Read the model definition and answer for the solid it produces. Units are mm, in the model's axes. Face numbers are marked on the shaded views. A direction names the side the tool comes from. Coordinates: 2 decimals unless noted, no trailing zeros. Loops run counter-clockwise (first coordinate to the right, second up) from the corner with the lowest first, then second, coordinate; pieces in that order, holes last. Notation, with made-up numbers: (42, -15.5) - (89, -15.5) arc R18 cw to (89, -4.5) - close; hole circle Ø3 at (39.5, 56). An arc over 180 degrees is marked (long way). Use one line per item in the form item = value. Start each with the question number.
1) A cutting plane is placed at A-A (y = 12.75). Give the vertices of the cut face in (x, z).
2) This flat-tipped pin is pushed along its axis until it touches: P1, Ø2, axis at x = -23, z = -9.5, coming from the +Y side. Where does it stop, or does it pass through?
3) Which of the six approach directions +Z, -Z, +X, -X, +Y, -Y give full straight-line access (tool end or side, diameter ignored) to the marked faces 1 and 2?
4) Consider line 1 (Z direction, x = -28, y = 13); line 2 (Y direction, x = -27.5, z = -4.5). Determine where each line is inside the solid, lowest interval first.
5) A cutting plane is placed at B-B (z = -35.5). Give the vertices of the cut face in (x, y).
6) A cutting plane is placed at C-C (x = -61). Give the vertices of the cut face in (y, z), and give its area (3 significant figures).
Autodesk Inventor part; units mm, degrees
ref_plane "YZ Plane" through (0, 0, 0) normal (1, 0, 0) x (0, 1, 0)
ref_plane "XZ Plane" through (0, 0, 0) normal (0, 1, 0) x (-1, 0, 0)
ref_plane "XY Plane" through (0, 0, 0) normal (0, 0, 1) x (1, 0, 0)
sketch "Sketch1" plane through (0, 0, 0) normal (0, 1, 0) x (-1, 0, 0)
  line L0 (0, 0) -> (74, 0)
  line L1 (74, 0) -> (74, -74)
  line L2 (74, -74) -> (0, -74)
  line L3 (0, -74) -> (0, 0)
  dimension "d0" = 74
  dimension "d1" = 74
extrude "Extrusion1" add sketch "Sketch1" along normal blind 10
sketch "Sketch2" plane through (0, 10, 0) normal (0, 1, 0) x (1, 0, 0)
  line L0 (0, 0) -> (0, 74)
  line L1 (0, 74) -> (-74, 74)
  line L2 (0, 0) -> (-74, 0)
  line L3 (-74, 0) -> (-74, 74)
  line L4 (-74, 74) -> (0, 74)
  line L5 (0, 74) -> (0, 0)
  line L6 (-72.5, 72.5) -> (-72.5, 1.5)
  line L7 (-72.5, 1.5) -> (-1.5, 1.5)
  line L8 (-1.5, 1.5) -> (-1.5, 72.5)
  line L9 (-1.5, 72.5) -> (-72.5, 72.5)
  dimension "d4" = 1.5
extrude "Extrusion2" add sketch "Sketch2" along normal blind 5
sketch "Sketch3" plane through (0, 0, 0) normal (0, -1, 0) x (1, 0, 0)
  line L0 (0, 0) -> (0, -74)
  line L1 (0, 0) -> (-74, 0)
  line L2 (-74, 0) -> (-74, -74)
  line L3 (-74, -74) -> (0, -74)
  line L4 (0, -74) -> (0, 0)
extrude "Extrusion3" cut sketch "Sketch3" against normal blind 5
sketch "Sketch4" plane through (0, 5, 0) normal (0, -1, 0) x (1, 0, 0)
  line L0 (0, 0) -> (0, -74)
  line L1 (-74, -74) -> (0, -74)
  line L2 (0, -74) -> (0, 0)
  line L3 (0, 0) -> (-74, 0)
  line L4 (-74, 0) -> (-74, -74)
extrude "Extrusion4" cut sketch "Sketch4" against normal blind 2
properties part number "DiffusorCapThin"
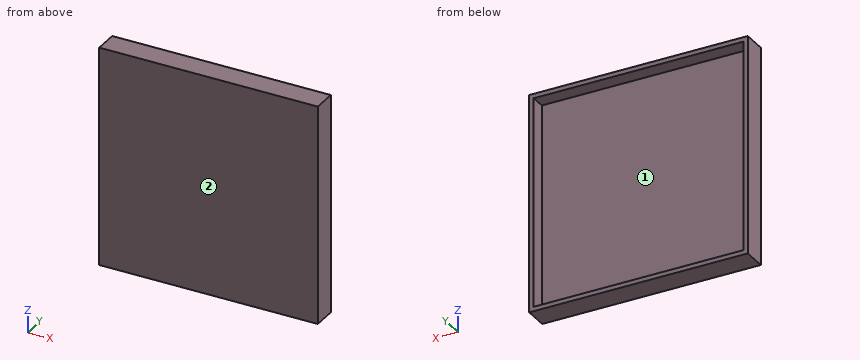
Found:
q1.outline = (-74, -74) - (0, -74) - (0, 0) - (-74, 0) - close; hole (-72.5, -72.5) - (-1.5, -72.5) - (-1.5, -1.5) - (-72.5, -1.5) - close
q2.P1 = 10
q3.face_1 = +Y
q3.face_2 = +Z, -Z, +X, -X, -Y
q4.line_1 = -74 to -72.5, -1.5 to 0
q4.line_2 = 7 to 10
q5.outline = (-74, 7) - (0, 7) - (0, 15) - (-1.5, 15) - (-1.5, 10) - (-72.5, 10) - (-72.5, 15) - (-74, 15) - close
q6.outline = (7, -74) - (15, -74) - (15, -72.5) - (10, -72.5) - (10, -1.5) - (15, -1.5) - (15, 0) - (7, 0) - close
q6.area = 237 mm^2
